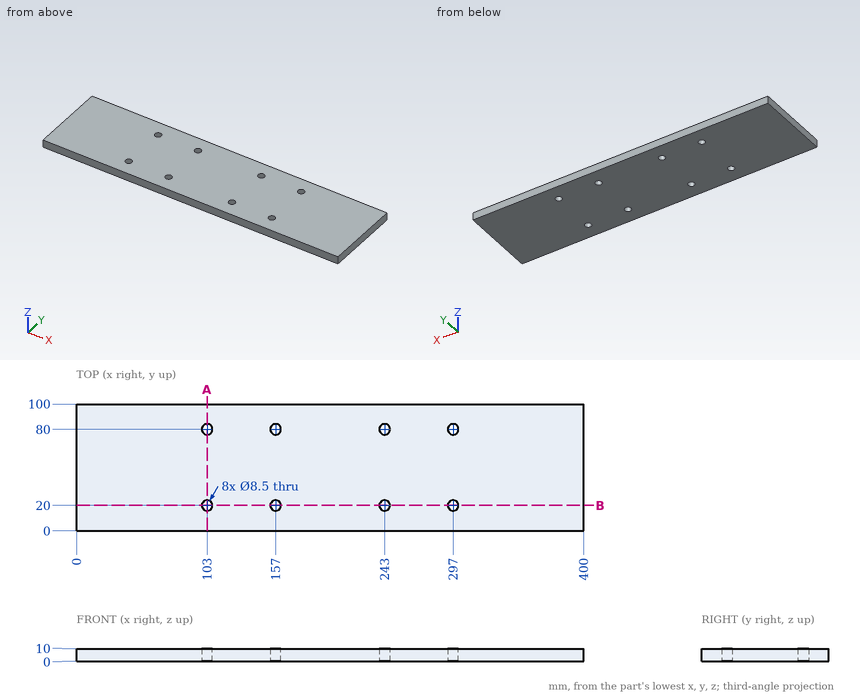
Source: three-view drawing plus pictorial views. Frame: mm from the lowest corner of the part. Coordinates: 2 decimals unless noted, no trailing zeros. Write each loop counter-clockwise with the first axis right and the second up, starting at its lowest first coordinate (ties: lowest second). Pieces come first, ordered by that corner, then holes. Notation, with made-up numbers: (29.5, -5) -> (47.5, -5) arc R22 cw to (47.5, 33) -> close; hole circle Ø10 at (12, 62). An arc over 180 degrees is marked (long way). Answer as a JSON object with one key per item and string values.
1. Section A-A on x = 103. Return the cut outline in (y, z), then the cut area to 3 significant figures.
Result set:
{"outline": "(0, 0) -> (15.75, 0) -> (15.75, 10) -> (0, 10) -> close; (24.25, 0) -> (75.75, 0) -> (75.75, 10) -> (24.25, 10) -> close; (84.25, 0) -> (100, 0) -> (100, 10) -> (84.25, 10) -> close", "area": "830 mm2"}
2. First-contact query: P1, Ø7, axis at x = 157, y = 80, coming from the +Z side; P2, Ø11, axis at x = 103, y = 80, coming from the -Z side. Flat tips, straight axial feed; report the tip coordinate or a pass-through.
Result set:
{"P1": "passes through", "P2": "stops at z = 0"}
3. Section B-B on y = 20. Return the cut outline in (x, z), then the cut area to 3 significant figures.
Result set:
{"outline": "(0, 0) -> (98.75, 0) -> (98.75, 10) -> (0, 10) -> close; (107.25, 0) -> (152.75, 0) -> (152.75, 10) -> (107.25, 10) -> close; (161.25, 0) -> (238.75, 0) -> (238.75, 10) -> (161.25, 10) -> close; (247.25, 0) -> (292.75, 0) -> (292.75, 10) -> (247.25, 10) -> close; (301.25, 0) -> (400, 0) -> (400, 10) -> (301.25, 10) -> close", "area": "3,660 mm2"}
4. Material intervals for line 1 (Y direction, x = 297, z = 6.5); line 2 (Y direction, x = 154, z = 4.25); line 3 (X direction, y = 79, z = 5.25), sorted ascending. Write a range as from..to.
Result set:
{"line 1": "y = 0..15.75, 24.25..75.75, 84.25..100", "line 2": "y = 0..16.99, 23.01..76.99, 83.01..100", "line 3": "x = 0..98.87, 107.13..152.87, 161.13..238.87, 247.13..292.87, 301.13..400"}
